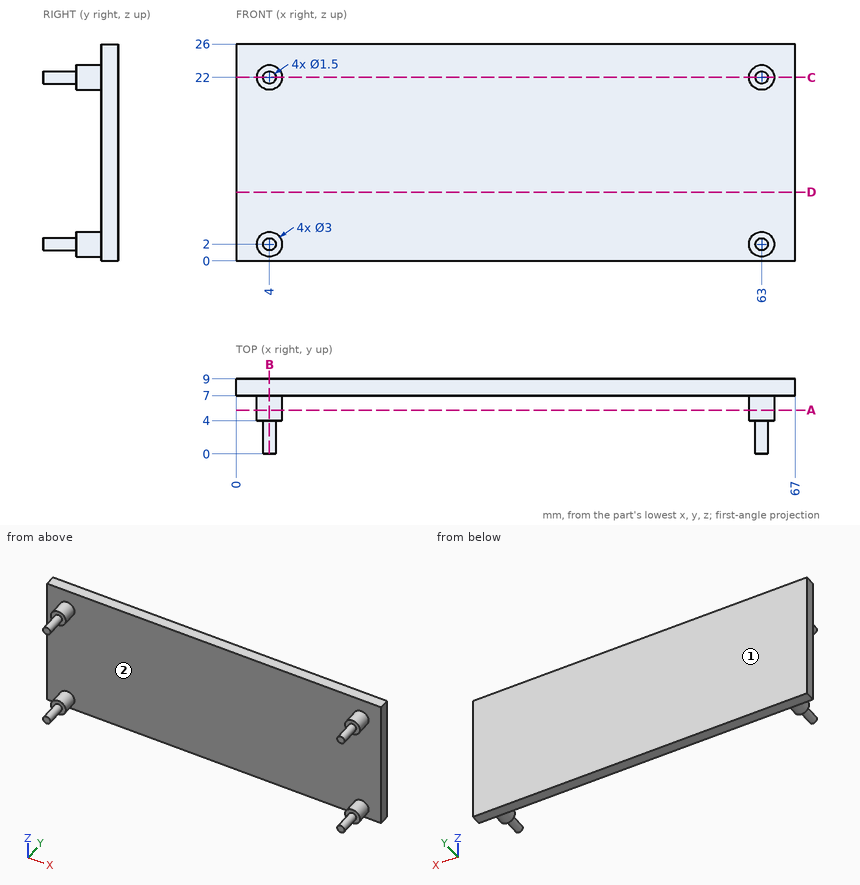
Print and shaded views of the part. All mm, measured from the part's lowest x, y and z. Round coordinates to 2 decimals unless told otherwise and drop trailing zeros. Write each loop counter-clockwise with the first axis right and the second up, starting at its lowest first coordinate (ties: lowest second). Pieces come first, ordered by that corner, then holes. Notation, with made-up numbers: (65.25, 78) -> (78.25, 78) arc R20 cw to (78.25, 113) -> close; hole circle Ø10 at (89.25, 18). An arc over 180 degrees is marked (long way). Answer in a Markdown table with one row per item. Add a question column.
Item 1: Saw through at A-A, the plane y = 5.25. Write the cut outline in (x, z).
Item 2: Saw through at B-B, the plane x = 4. Write the cut outline in (y, z), then the cut area to 3 significant figures.
Item 3: Drill centre lines: line 1 (Y direction, x = 57, z = 8.5); line 2 (X direction, y = 6.25, z = 21.5); line 3 (Z direction, x = 4, y = 3.25). Where is each one in solid material? Low to high. Write a range as from..to.
Item 4: Saw through at C-C, the plane z = 22. Write the cut outline in (x, y).
Item 5: Mould opens along X. For the marked faces 1 and 2 say: pulls with the +X half, pulls with the -X half, needs draft (parallel to the pull), parting line crosses it, or undercut.
Item 6: Drop flat-ended pins along their axis: pin 1 Ø4 at (y, z) = (3, 17) entering from -X; pin 2 Ø8 at (x, z) = (28.5, 8) entering from -Y. Give the stop position or say it passes through.
Item 7: Saw through at D-D, the plane z = 8.25. Write the cut outline in (x, y), then the cut area to 3 significant figures.
Findings below:
| question | item | result |
|---|---|---|
| 1 | outline | circle Ø3 at (4, 2); circle Ø3 at (4, 22); circle Ø3 at (63, 2); circle Ø3 at (63, 22) |
| 2 | outline | (0, 1.25) -> (4, 1.25) -> (4, 0.5) -> (7, 0.5) -> (7, 0) -> (9, 0) -> (9, 26) -> (7, 26) -> (7, 23.5) -> (4, 23.5) -> (4, 22.75) -> (0, 22.75) -> (0, 21.25) -> (4, 21.25) -> (4, 20.5) -> (7, 20.5) -> (7, 3.5) -> (4, 3.5) -> (4, 2.75) -> (0, 2.75) -> close |
| 2 | area | 82.0 mm^2 |
| 3 | line 1 | y = 7..9 |
| 3 | line 2 | x = 2.59..5.41, 61.59..64.41 |
| 3 | line 3 | z = 1.25..2.75, 21.25..22.75 |
| 4 | outline | (0, 7) -> (2.5, 7) -> (2.5, 4) -> (3.25, 4) -> (3.25, 0) -> (4.75, 0) -> (4.75, 4) -> (5.5, 4) -> (5.5, 7) -> (61.5, 7) -> (61.5, 4) -> (62.25, 4) -> (62.25, 0) -> (63.75, 0) -> (63.75, 4) -> (64.5, 4) -> (64.5, 7) -> (67, 7) -> (67, 9) -> (0, 9) -> close |
| 5 | face 1 | needs draft |
| 5 | face 2 | undercut |
| 6 | pin 1 | passes through |
| 6 | pin 2 | stops at y = 7 |
| 7 | outline | (0, 7) -> (67, 7) -> (67, 9) -> (0, 9) -> close |
| 7 | area | 134 mm^2 |
